```python
from build123d import *

# Parameters (mm, degrees)
SKETCH1_W            = 75
SKETCH1_H            = 93.5
BOSS_EXTRUDE1_DEPTH  = 3
SKETCH2_R            = 3.1
CUT_EXTRUDE1_DEPTH   = 61.006770451
LPATTERN1_COUNT      = 2
LPATTERN1_PITCH      = 64
LPATTERN1_COUNT_DIR2 = 2
LPATTERN1_PITCH_DIR2 = 64
SKETCH3_W            = 38
SKETCH3_H            = 12
CUT_EXTRUDE2_DEPTH   = 61.006770451


with BuildPart() as part:
    # Sketch1 → Boss-Extrude1 (new body)
    with BuildSketch(Plane.XY):
        Rectangle(SKETCH1_W, SKETCH1_H)
    extrude(amount=BOSS_EXTRUDE1_DEPTH)

    # Sketch2 → Cut-Extrude1 (cut, through all)
    with BuildSketch(Plane.XY.offset(3)):
        with Locations((-32, 32)):
            Circle(SKETCH2_R)
    cut_extrude1 = extrude(amount=-CUT_EXTRUDE1_DEPTH, mode=Mode.SUBTRACT)

    # LPattern1: Cut-Extrude1 2 × 2
    with Locations(*[(i * LPATTERN1_PITCH, -j * LPATTERN1_PITCH_DIR2, 0) for i in range(LPATTERN1_COUNT) for j in range(LPATTERN1_COUNT_DIR2) if (i, j) != (0, 0)]):
        add(cut_extrude1, mode=Mode.SUBTRACT)

    # Sketch3 → Cut-Extrude2 (cut, through all)
    with BuildSketch(Plane.XY.offset(3)):
        with Locations((0, 40.75)):
            Rectangle(SKETCH3_W, SKETCH3_H)
    extrude(amount=-CUT_EXTRUDE2_DEPTH, mode=Mode.SUBTRACT)


solid = part.part
```
Could you check a few things on this model? Use its own coordinates, in mm. A direction names the side the tool comes from. Coordinates: 2 decimals unless noted, no trailing zeros. Order: outer loops, then holes, each group sorted by start corner. A loop starts at its lowest first (then second) coordinate and runs counter-clockwise, first axis right, second up. Notation, with made-up numbers: M -37.75,77 L 14.25,77 A30 cw 14.25,113 Z; hole C 69.5,50 d6. An arc over 180 degrees is marked long. Use one line per item in the form item = value. Start each with the question number.
1. Suppose I cut it at D-D on z = 0.7. Write out the boundary of the cut face in (x, y).
2. Please list where these lines run through material, in increasing order: line 1 (Y direction, x = -32, z = 1.65); line 2 (Y direction, x = -11, z = 0.5); line 3 (X direction, y = 34, z = 1.25).
3. Suppose I cut it at B-B on y = 37. Write out the boundary of the cut face in (x, z).
4. On a 3-axis mill with a long thin cutter (end or side, diameter ignored), from which of +Z, -Z, +X, -X, +Y, -Y can I reach the whole of each face in a straight line? I mean faces 1 (the cylindrical face through (29.72, -29.9, 1.52)), 2 (the flat face through (-19, 41, 2)). Say none if no direction works.
5. We'd pull the mould along Y, two halves only. Please class faces 3 (the cylindrical face through (29.72, 34.1, 1.52)), 4 (the flat face through (37.5, -1, 1)), 5 (the flat face through (0, 34.75, 2)): +Y half, -Y half, draft (parallel to the pull), parting line (faces both ways), or undercut.
6. Suppose I cut it at C-C on y = -32. Write out the boundary of the cut face in (x, z).
7. Suppose I cut it at A-A on x = 32. Write out the boundary of the cut face in (y, z).
8. For pin 1 (3.5 mm diameter, centred on x = -32, y = 32, fed in from +Z); pin 2 (0.9 mm diameter, centred on x = 5.5, z = 2, fed in from +Y), each with a flat end and sliding along its axis, tell me the tip position at first contact or that it passes through.
Geometry says:
q1.outline = M -37.5,-46.75 L 37.5,-46.75 L 37.5,46.75 L 19,46.75 L 19,34.75 L -19,34.75 L -19,46.75 L -37.5,46.75 Z; hole C -32,-32 d6.2; hole C -32,32 d6.2; hole C 32,-32 d6.2; hole C 32,32 d6.2
q2.line_1 = -46.75 to -35.1, -28.9 to 28.9, 35.1 to 46.75
q2.line_2 = -46.75 to 34.75
q2.line_3 = -37.5 to -34.37, -29.63 to 29.63, 34.37 to 37.5
q3.outline = M -37.5,0 L -19,0 L -19,3 L -37.5,3 Z; M 19,0 L 37.5,0 L 37.5,3 L 19,3 Z
q4.face_1 = +Z, -Z
q4.face_2 = +Z, -Z, +Y
q5.face_3 = undercut
q5.face_4 = draft
q5.face_5 = +Y half
q6.outline = M -37.5,0 L -35.1,0 L -35.1,3 L -37.5,3 Z; M -28.9,0 L 28.9,0 L 28.9,3 L -28.9,3 Z; M 35.1,0 L 37.5,0 L 37.5,3 L 35.1,3 Z
q7.outline = M -46.75,0 L -35.1,0 L -35.1,3 L -46.75,3 Z; M -28.9,0 L 28.9,0 L 28.9,3 L -28.9,3 Z; M 35.1,0 L 46.75,0 L 46.75,3 L 35.1,3 Z
q8.pin_1 = through
q8.pin_2 = 34.75
